Could you check a few things on this model? Use its own coordinates, in mm. Face numbers are marked on the shaded views. Give positions to 0.01 mm unless a question says otherwise; leave off trailing zeros. Order: outer loops, then holes, each group sorted by start corner. A loop starts at its lowest first (then second) coordinate and runs counter-clockwise, first axis right, second up.
Autodesk Inventor part; units mm, degrees
ref_plane "YZ Plane" through (0, 0, 0) normal (1, 0, 0) x (0, 1, 0)
ref_plane "XZ Plane" through (0, 0, 0) normal (0, 1, 0) x (-1, 0, 0)
ref_plane "XY Plane" through (0, 0, 0) normal (0, 0, 1) x (1, 0, 0)
sketch "Sketch1" plane through (0, 0, 0) normal (0, 1, 0) x (-1, 0, 0)
  line L0 (0, 0) -> (-139.7, 0)
  line L1 (-107.95, -101.6) -> (0, -101.6)
  line L2 (0, -101.6) -> (0, 0)
  line L3 (-107.95, -101.6) -> (-139.7, -50.8)
  line L4 (-139.7, -50.8) -> (-139.7, 0)
  circle A0 centre (-25.4, -63.5) radius 12.7
  circle A1 centre (-76.2, -38.1) radius 12.7
  dimension "d0" = 50.8
  dimension "d1" = 101.6
  dimension "d2" = 107.95
  dimension "d3" = 139.7
  dimension "d5" = 25.4
  dimension "d6" = 63.5
  dimension "d7" = 38.1
  dimension "d8" = 76.2
  dimension "d9" = 25.4
extrude "Extrusion1" add sketch "Sketch1" along normal blind 6.35
sketch "Sketch2" plane through (0, 6.35, 0) normal (0, 1, 0) x (1, 0, 0)
  circle A0 centre (76.2, 38.1) radius 12.7
  point P0 (0, 0)
hole "Hole1" at (76.2, 6.35, -38.1) direction (0, -1, 0) diameter 25.4 end through all counterbore diameter 50.8 counterbore depth 3.175
properties part number "GuidePlate"
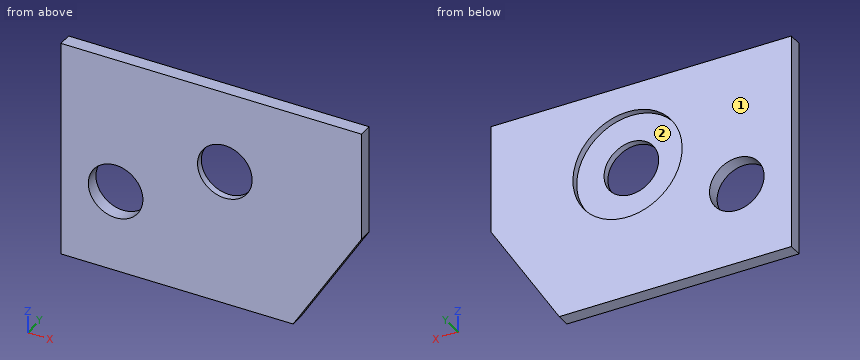
Item 1: Imagine slicing it at A-A on x = 76.2. List the corners of the cut face in (y, z) for me (3 decimals), then the cut area to 3 significant figures.
Findings:
outline: (0, -101.6) - (6.35, -101.6) - (6.35, -63.5) - (3.175, -63.5) - (3.175, -50.8) - (0, -50.8) - close; (0, -25.4) - (3.175, -25.4) - (3.175, -12.7) - (6.35, -12.7) - (6.35, 0) - (0, 0) - close
area: 403 mm2
Item 2: Imagine slicing it at B-B on y = 1.75. List the corners of the cut face in (x, z) for me, then the cut area to 3 significant figures.
Findings:
outline: (0, -101.6) - (107.95, -101.6) - (139.7, -50.8) - (139.7, 0) - (0, 0) - close; hole circle Ø25.4 at (25.4, -63.5); hole circle Ø25.4 at (76.2, -38.1)
area: 12,400 mm2
Item 3: Please list where these lines run through material, in increasing order: line 1 along X through (y, z) = (4.3, -38.1); line 2 along Z through (x, y) = (25.4, 2); line 3 along Z through (x, y) = (76.2, 1.15).
Findings:
line 1: x = 0 to 50.8, 101.6 to 139.7
line 2: z = -101.6 to -76.2, -50.8 to 0
line 3: z = -101.6 to -50.8, -25.4 to 0
Item 4: Imagine slicing it at D-D on x = 25.4. List the corners of the cut face in (y, z) for me.
Findings:
outline: (0, -101.6) - (6.35, -101.6) - (6.35, -76.2) - (0, -76.2) - close; (0, -50.8) - (6.35, -50.8) - (6.35, 0) - (0, 0) - close
Item 5: Imagine slicing it at C-C on z = -38.1. List the corners of the cut face in (x, y) for me (3 decimals), then the cut area to 3 significant figures.
Findings:
outline: (0, 0) - (63.5, 0) - (63.5, 3.175) - (50.8, 3.175) - (50.8, 6.35) - (0, 6.35) - close; (88.9, 0) - (139.7, 0) - (139.7, 6.35) - (101.6, 6.35) - (101.6, 3.175) - (88.9, 3.175) - close
area: 645 mm2
Item 6: We'd pull the mould along X, two halves only. Please class the marked faces 1 and 2: +X half, -X half, draft (parallel to the pull), parting line (faces both ways), or undercut.
Findings:
face 1: draft
face 2: undercut
Item 7: For pin 1 (1.5 mm diameter, centred on x = 80, z = -21.5, fed in from +Y) (3 decimals), with a flat end and sliding along its axis, tell me the tip position at first contact or that it passes through.
Findings:
pin 1: stops at y = 3.175
